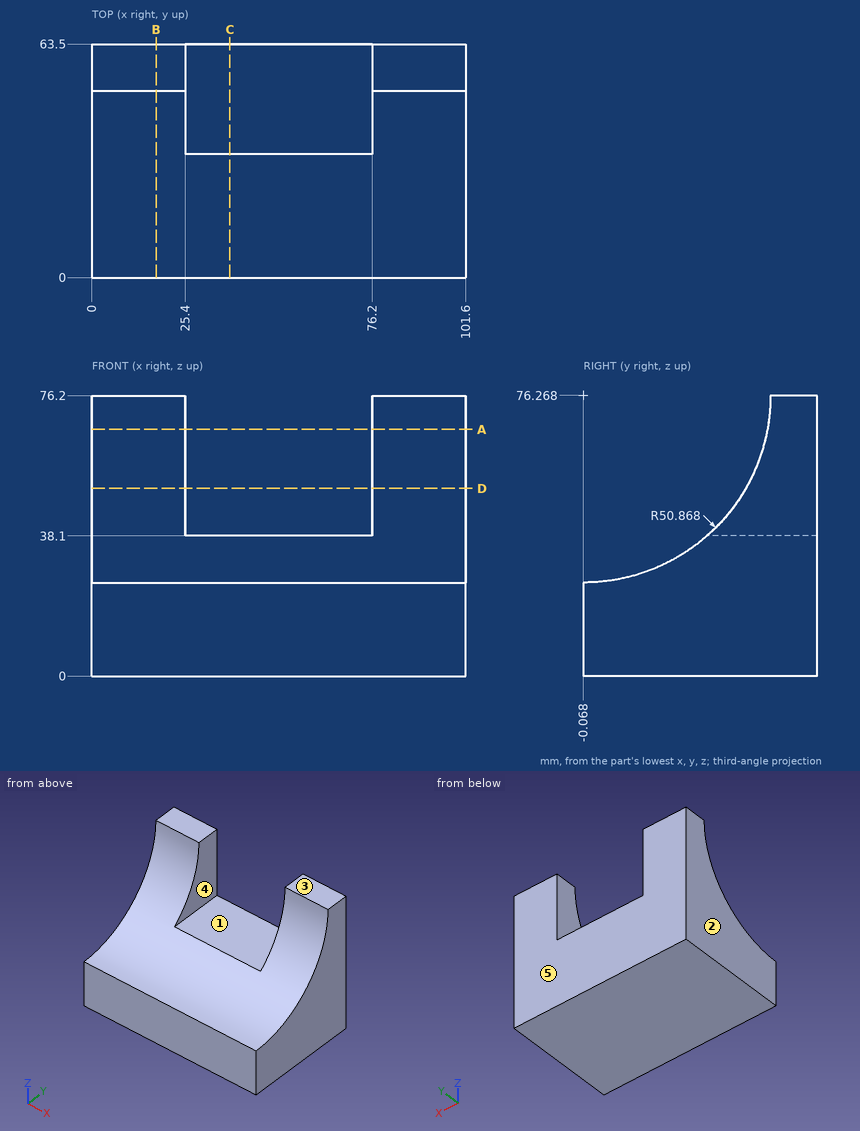
Here's the drawing with two shaded views (mm, measured from the low corner). I have some questions. A direction names the side the tool comes from. Give positions to 0.01 mm unless a question says otherwise; leave off trailing zeros. Loops run counter-clockwise (first coordinate to the right, second up) from the corner with the lowest first, then second, coordinate; pieces in that order, holes last. Notation, with made-up numbers: M 77.25,56.25 L 111.25,56.25 A17 ccw 111.25,74.25 Z; hole C 87.25,-3 d9. An arc over 180 degrees is marked long. One line per item, written item: value.
(1) Suppose I cut it at C-C on x = 37.5. List the corners of the cut face in (y, z) for me, plus the area to 3 significant figures.
Returned:
outline: M 0,0 L 63.5,0 L 63.5,38.1 L 33.56,38.1 A50.87 cw 0,25.4 Z
area: 2,130 mm^2
(2) Which directions (+Z, -Z, +X, -X, +Y, -Y) give clear straight access to the entire face, cutting with the end or side of a thin tool? Please do the marked faces 4 and 5.
Returned:
face 4: +Z, +Y, -Y
face 5: +Z, -Z, +X, -X, +Y
(3) Will these pins go through, and if not, where does the flat tip stop? pin 1 (1 mm diameter, centred on x = 20.5, z = 52.5, fed in from -Y); pin 2 (12 mm diameter, centred on x = 20, z = 42, fed in from -Y); pin 3 (6 mm diameter, centred on x = 64, y = 26, fed in from +Z).
Returned:
pin 1: y = 44.64
pin 2: y = 31.01
pin 3: z = 34.52
(4) I need wall thicknesses on line 1 (X direction, y = 50, z = 40); line 2 (Z direction, x = 39, y = 53); line 3 (Z direction, x = 36, y = 13). Which ranges of each line are inside material? Lowest first, please.
Returned:
line 1: 0 to 25.4, 76.2 to 101.6
line 2: 0 to 38.1
line 3: 0 to 27.11
(5) Suppose I cut it at B-B on x = 17.5. List the corners of the cut face in (y, z) for me.
Returned:
outline: M 0,0 L 63.5,0 L 63.5,76.2 L 50.8,76.2 A50.87 cw 0,25.4 Z
(6) Suppose I cut it at D-D on z = 51. List the corners of the cut face in (x, y) for me.
Returned:
outline: M 0,44.08 L 25.4,44.08 L 25.4,63.5 L 0,63.5 Z; M 76.2,44.08 L 101.6,44.08 L 101.6,63.5 L 76.2,63.5 Z
(7) Suppose I cut it at A-A on z = 67. List the corners of the cut face in (x, y) for me.
Returned:
outline: M 0,49.95 L 25.4,49.95 L 25.4,63.5 L 0,63.5 Z; M 76.2,49.95 L 101.6,49.95 L 101.6,63.5 L 76.2,63.5 Z
(8) We'd pull the mould along X, two halves only. Please class the marked faces 1, 2 and 3: released by +X, released by -X, zero draft, split by the parting line, or undercut.
Returned:
face 1: undercut
face 2: released by -X
face 3: zero draft
